Autodesk Fusion 360 part; units mm, degrees
sketch "Sketch1" plane through (0, 0, 0) normal (0, 0, 1) x (1, 0, 0)
  line L0 (-180, 122) -> (180, 122)
  line L1 (180, 122) -> (180, -122)
  line L2 (180, -122) -> (-180, -122)
  line L3 (-180, -122) -> (-180, 122)
  line L4 (-180, 122) -> (180, -122) construction
  line L5 (180, 122) -> (-180, -122) construction
  line L6 (-150, 100) -> (150, 100)
  line L7 (150, 100) -> (150, -100)
  line L8 (150, -100) -> (-150, -100)
  line L9 (-150, -100) -> (-150, 100)
  line L10 (-150, 100) -> (150, -100) construction
  line L11 (150, 100) -> (-150, -100) construction
  dimension "d1" = 244
  dimension "d2" = 360
  dimension "d3" = 300
  dimension "d4" = 200
extrude "Extrude1" add sketch "Sketch1" along normal blind 3
extrude "Extrude2" add 1 faces at (-150, -33.3333, 1) along direction (1, 0, 0) blind 30
extrude "Extrude3" add 1 faces at (150, 33.3333, 1) along direction (-1, 0, 0) blind 30
sketch "Sketch2" plane through (0, 0, 3) normal (0, 0, 1) x (-1, 0, 0)
  line L0 (-120, 100) -> (120, 100)
  line L1 (120, 100) -> (120, -100)
  line L2 (120, -100) -> (-120, -100)
  line L3 (-120, -100) -> (-120, 100)
  line L4 (180, 122) -> (-180, 122)
  line L5 (-180, 122) -> (-180, -122)
  line L6 (-180, -122) -> (180, -122)
  line L7 (180, -122) -> (180, 122)
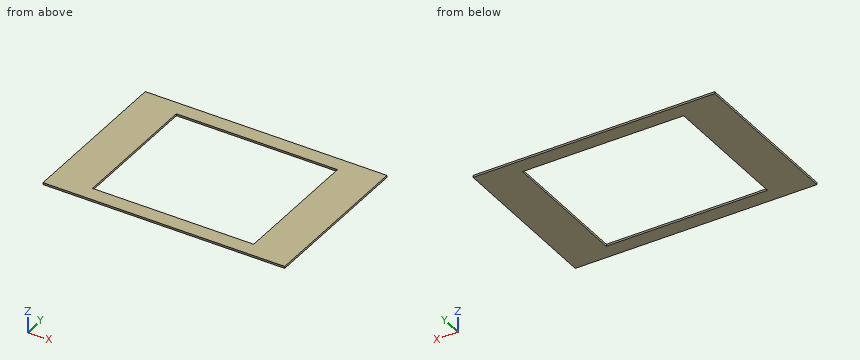
Read the model definition and answer for the solid it produces. Units are mm, in the model's axes. Give positions to 0.01 mm unless a question says otherwise; leave off trailing zeros. Loops run counter-clockwise (first coordinate to the right, second up) from the corner with the lowest first, then second, coordinate; pieces in that order, holes last. Notation, with made-up numbers: (71, 35) - (113, 35) arc R22 ccw to (113, 47) - close; hole circle Ø5 at (51.25, 89.25). An arc over 180 degrees is marked (long way). Answer as CSV lines item,"result". Start each with the question number.
1) Find section C-C (x = 108.5). Write down the section's boundary in (y, z).
2) Find section A-A (z = 0.5). Write down the section's boundary in (x, y), then the cut area to 3 significant figures.
3) This flat-tipped pin is pushed along its axis until it touches: pin 1 Ø3 at (x, y) = (138, 74) entering from -Z. Where does it stop, or does it pass through?
4) Straight lines are drawn through the part: L1, parallel to X at y = 44, z = 0.55; L2, parallel to Y at x = 84.5, z = 1.1. For each, find the intervals that lie inside material, in ascending order. Write a range as from..to.
5) Find section B-B (y = 75). Write down the section's boundary in (x, z).
Findings below:
1,outline,"(-122, 0) - (-100, 0) - (-100, 3) - (-122, 3) - close; (100, 0) - (122, 0) - (122, 3) - (100, 3) - close"
2,outline,"(-180, -122) - (180, -122) - (180, 122) - (-180, 122) - close; hole (-120, -100) - (120, -100) - (120, 100) - (-120, 100) - close"
2,area,"39,800 mm^2"
3,pin 1,"z = 0"
4,L1,"-180..-120, 120..180"
4,L2,"-122..-100, 100..122"
5,outline,"(-180, 0) - (-120, 0) - (-120, 3) - (-180, 3) - close; (120, 0) - (180, 0) - (180, 3) - (120, 3) - close"
